The listing builds one solid part. Answer for the finished solid, in the listing's coordinates (mm). Coordinates: 2 decimals unless noted, no trailing zeros. Write each loop counter-clockwise with the first axis right and the second up, starting at its lowest first coordinate (ties: lowest second). Pieces come first, ordered by that corner, then holes.
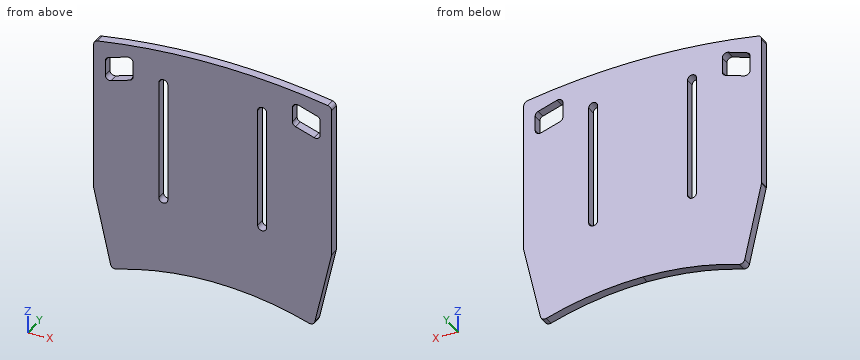
from build123d import *

# Parameters (mm, degrees)
RESSALTO_EXTRUS_O1_DEPTH = 2


with BuildPart() as part:
    # Esboço1 → Ressalto-extrusão1 (new body)
    with BuildSketch(Plane(origin=(0, 0, 0), x_dir=(1, 0, 0), z_dir=(0, 1, 0))):
        with BuildLine():
            Line((-22.739996026, 26.420017885), (-26.47618706, 9.607158229))
            ThreePointArc((-26.47618706, 9.607158229), (-26.494028938, 9.499344543), (-26.5, 9.390227771))
            Line((-26.5, 9.390227771), (-26.5, -24.299313819))
            ThreePointArc((-26.5, -24.299313819), (-26.265286485, -24.943003648), (-25.671326807, -25.284528072))
            ThreePointArc((-25.671326807, -25.284528072), (0, -27.5), (25.671326807, -25.284528072))
            ThreePointArc((25.671326807, -25.284528072), (26.265286485, -24.943003648), (26.5, -24.299313819))
            Line((26.5, -24.299313819), (26.5, 9.607158229))
            Line((26.5, 9.607158229), (22.763808965, 26.420017885))
            ThreePointArc((22.763808965, 26.420017885), (22.284676967, 27.070806428), (21.480921688, 27.154893592))
            ThreePointArc((21.480921688, 27.154893592), (10.878133716, 24.629860221), (0.01190647, 23.781325176))
            ThreePointArc((0.01190647, 23.781325176), (-10.854320777, 24.629860221), (-21.457108748, 27.154893592))
            ThreePointArc((-21.457108748, 27.154893592), (-22.260864027, 27.070806428), (-22.739996026, 26.420017885))
        make_face()
        with BuildLine():
            Line((23.945153985, -17.77729625), (23.945153985, -21.127458538))
            ThreePointArc((23.945153985, -21.127458538), (23.754375079, -21.714962769), (23.254831543, -22.07830017))
            Line((23.254831543, -22.07830017), (19.076176544, -23.439237296))
            ThreePointArc((19.076176544, -23.439237296), (18.178994755, -23.297616757), (17.766498985, -22.488395663))
            Line((17.766498985, -22.488395663), (17.766498985, -19.138233375))
            ThreePointArc((17.766498985, -19.138233375), (17.957277891, -18.550729144), (18.456821427, -18.187391742))
            Line((18.456821427, -18.187391742), (22.635476426, -16.826454617))
            ThreePointArc((22.635476426, -16.826454617), (23.532658215, -16.968075156), (23.945153985, -17.77729625))
        make_face(mode=Mode.SUBTRACT)
        with BuildLine():
            Line((-10, 7.500138791), (-10, -19.499861209))
            ThreePointArc((-10, -19.499861209), (-11, -20.499861209), (-12, -19.499861209))
            Line((-12, -19.499861209), (-12, 7.500138791))
            ThreePointArc((-12, 7.500138791), (-11, 8.500138791), (-10, 7.500138791))
        make_face(mode=Mode.SUBTRACT)
        with BuildLine():
            Line((-23.231018603, -22.07830017), (-19.052363604, -23.439237296))
            ThreePointArc((-19.052363604, -23.439237296), (-18.155181815, -23.297616757), (-17.742686046, -22.488395663))
            Line((-17.742686046, -22.488395663), (-17.742686046, -19.138233375))
            ThreePointArc((-17.742686046, -19.138233375), (-17.933464951, -18.550729144), (-18.433008487, -18.187391742))
            Line((-18.433008487, -18.187391742), (-22.611663487, -16.826454617))
            ThreePointArc((-22.611663487, -16.826454617), (-23.508845275, -16.968075156), (-23.921341045, -17.77729625))
            Line((-23.921341045, -17.77729625), (-23.921341045, -21.127458538))
            ThreePointArc((-23.921341045, -21.127458538), (-23.730562139, -21.714962769), (-23.231018603, -22.07830017))
        make_face(mode=Mode.SUBTRACT)
        with BuildLine():
            Line((10.02381294, 7.500138791), (10.02381294, -19.499861209))
            ThreePointArc((10.02381294, -19.499861209), (11.02381294, -20.499861209), (12.02381294, -19.499861209))
            Line((12.02381294, -19.499861209), (12.02381294, 7.500138791))
            ThreePointArc((12.02381294, 7.500138791), (11.02381294, 8.500138791), (10.02381294, 7.500138791))
        make_face(mode=Mode.SUBTRACT)
    extrude(amount=RESSALTO_EXTRUS_O1_DEPTH)


solid = part.part
1. Find the intervals of material crossed by L1, parallel to X at y = 1.6, z = 16.5; L2, parallel to X at y = 1.55, z = 19; L3, parallel to Z at x = 0.5, y = 0.7, in increasing order.
Results found:
L1: x = -26.5 to -12, -10 to 10.02, 12.02 to 26.5
L2: x = -26.5 to -23.92, -17.75 to -12, -10 to 10.02, 12.02 to 17.78, 23.95 to 26.5
L3: z = -23.78 to 27.5
2. Section C-C on y = 0.85 is taken. State how many separate pieces and enclosed holes the cut face has, then the cut area to 3 significant figures.
Results found:
separate pieces: 1
enclosed holes: 4
area: 2,510 mm2
3. Section D-D on z = -18 is taken. Give the vertices of the cut face in (x, y), then the cut area to 3 significant figures.
Results found:
outline: (-24.61, 0) - (24.63, 0) - (24.63, 2) - (-24.61, 2) - close
area: 98.5 mm2
4. Section B-B on x = -11 is taken. Give the vertices of the cut face in (y, z).
Results found:
outline: (0, -24.65) - (2, -24.65) - (2, -8.5) - (0, -8.5) - close; (0, 20.5) - (2, 20.5) - (2, 27.1) - (0, 27.1) - close
5. Section A-A on z = 15.5 is taken. Give the vertices of the cut face in (x, y).
Results found:
outline: (-26.5, 0) - (-12, 0) - (-12, 2) - (-26.5, 2) - close; (-10, 0) - (10.02, 0) - (10.02, 2) - (-10, 2) - close; (12.02, 0) - (26.5, 0) - (26.5, 2) - (12.02, 2) - close
6. Flat-ended cylindrical pins translate along their axes: P1, Ø1, axis at y = 1.5, z = -10.5, coming from the -X side; P2, Ø1, axis at x = -18, y = 1, coming from the +Z side. Find the tip coordinate at first contact, or state that the pin passes through.
Results found:
P1: stops at x = -26.39
P2: stops at z = 26.47
